Can you work these out from the model? Positions are in its coordinate system, mm. A direction names the side the tool comes from. Coordinates: 2 decimals unless noted, no trailing zeros. Order: outer loops, then holes, each group sorted by start corner. A loop starts at its lowest first (then second) coordinate and runs counter-clockwise, first axis right, second up. Notation, with made-up numbers: (63.25, 65) -> (76.25, 65) arc R30 cw to (76.25, 87) -> close; hole circle Ø3 at (39.5, -8). An arc over 180 degrees is marked (long way). Answer as CSV lines item,"result".
from build123d import *

# Parameters (mm, degrees)
SKETCH_1_W          = 60
SKETCH_1_H          = 5
EXTRUDE_1_DEPTH     = 3.18
SKETCH_2_R          = 4
EXTRUDE_2_DEPTH     = 3.18
SKETCH_3_R          = 2.395
CUT_EXTRUDE_1_DEPTH = 3.18
FILLET_3_R          = 8
FILLET_4_R          = 8
FILLET_5_R          = 8


with BuildPart() as part:
    # 草图1 → 凸台-拉伸1 (new body)
    with BuildSketch(Plane(origin=(0, 0, 0), x_dir=(1, 0, 0), z_dir=(0, 1, 0))):
        Rectangle(SKETCH_1_W, SKETCH_1_H)
    extrude(amount=EXTRUDE_1_DEPTH)

    # 草图2 → 凸台-拉伸2 (add)
    with BuildSketch(Plane(origin=(0, 0, 0), x_dir=(1, 0, 0), z_dir=(0, 1, 0))):
        with Locations((30, 0)):
            Circle(SKETCH_2_R)
        with Locations((-30, 0)):
            Circle(SKETCH_2_R)
    extrude(amount=EXTRUDE_2_DEPTH)

    # 草图3 → 切除-拉伸1 (cut)
    with BuildSketch(Plane(origin=(0, 0, 0), x_dir=(1, 0, 0), z_dir=(0, 1, 0))):
        with Locations(Location((30, 0, 0), (0, 0, 270))):
            Circle(SKETCH_3_R)
        with Locations(Location((-30, 0, 0), (0, 0, 270))):
            Circle(SKETCH_3_R)
    extrude(amount=CUT_EXTRUDE_1_DEPTH, mode=Mode.SUBTRACT)

    # 圆角3
    fillet_3_edges = [part.edges().sort_by_distance(p)[0] for p in [
        (-26.877501001, 1.59, -2.5),
    ]]
    fillet(fillet_3_edges, radius=FILLET_3_R)

    # 圆角4
    fillet_4_edges = [part.edges().sort_by_distance(p)[0] for p in [
        (-26.877501001, 1.59, 2.5),
    ]]
    fillet(fillet_4_edges, radius=FILLET_4_R)

    # 圆角5
    fillet_5_edges = [part.edges().sort_by_distance(p)[0] for p in [
        (26.877501001, 1.59, -2.5),
        (26.877501001, 1.59, 2.5),
    ]]
    fillet(fillet_5_edges, radius=FILLET_5_R)


solid = part.part
Q1. Imagine slicing it at A-A (x = -30). List the corners of the cut face in (y, z) for me (3 decimals).
Solution:
outline,"(0, -4) -> (3.18, -4) -> (3.18, -2.395) -> (0, -2.395) -> close; (0, 2.395) -> (3.18, 2.395) -> (3.18, 4) -> (0, 4) -> close"
Q2. Which directions (+Z, -Z, +X, -X, +Y, -Y) give clear straight access to the entire face, cutting with the end or side of a thin tool? Please do faces 4 (the cylindrical face through (-32.338, 1.568, -0.519)), 5 (the cylindrical face through (-26.163, 1.568, -2.747)), 6 (the flat face through (0, 2, 2.5)).
Solution:
face 4,"+Y, -Y"
face 5,"-Z, +Y, -Y"
face 6,"+Z, +Y, -Y"
Q3. Imagine slicing it at B-B (y = 2.35). List the corners of the cut face in (x, z) for me (1 decimal), and give its area (3 significant figures).
Solution:
outline,"(-28.1, -3.5) arc R8 cw to (-24.2, -2.5) -> (24.2, -2.5) arc R8 cw to (28.1, -3.5) arc R4 ccw (long way) to (28.1, 3.5) arc R8 cw to (24.2, 2.5) -> (-24.2, 2.5) arc R8 cw to (-28.1, 3.5) arc R4 ccw (long way) to start; hole circle Ø4.8 at (-30, 0); hole circle Ø4.8 at (30, 0)"
area,"330 mm2"
Q4. We'd pull the mould along Z, two halves only. Please class faces 1 (the cylindrical face through (32.02, 1.57, 1.29)), 2 (the cylindrical face through (-34, 2, 0)), 3 (the flat face through (0, 3.18, 0)): pulls with the +Z half, pulls with the -Z half, needs draft (parallel to the pull), parting line crosses it, or undercut.
Solution:
face 1,"undercut"
face 2,"parting line crosses it"
face 3,"needs draft"
Q5. Imagine slicing it at C-C (z = 0). List the corners of the cut face in (x, y) for me (3 decimals), and give its area (3 significant figures).
Solution:
outline,"(-34, 0) -> (-32.395, 0) -> (-32.395, 3.18) -> (-34, 3.18) -> close; (-27.605, 0) -> (27.605, 0) -> (27.605, 3.18) -> (-27.605, 3.18) -> close; (32.395, 0) -> (34, 0) -> (34, 3.18) -> (32.395, 3.18) -> close"
area,"186 mm2"
Q6. Imagine slicing it at D-D (x = 1). List the corners of the cut face in (y, z) for me.
Solution:
outline,"(0, -2.5) -> (3.18, -2.5) -> (3.18, 2.5) -> (0, 2.5) -> close"
Q7. If I drill on line 1 (X direction, y = 2.1, z = 0) (3 decimals); line 2 (X direction, y = 2.3, z = 1.25); line 3 (Z direction, x = -22.5, y = 2.6), over which ranges is the centre line in solid material (lowest first)?
Solution:
line 1,"-34 to -32.395, -27.605 to 27.605, 32.395 to 34"
line 2,"-33.8 to -32.04, -27.96 to 27.96, 32.04 to 33.8"
line 3,"-2.5 to 2.5"
Q8. For P1, Ø1.6, axis at x = 7, y = 2, coming from the +Z side; P2, Ø1.6, axis at x = 4, y = 2.5, coming from the -Z side, each with a flat end and sliding along its axis, tell me the tip position at first contact or that it passes through.
Solution:
P1,"z = 2.5"
P2,"z = -2.5"
